```python
from build123d import *
from build123d.topology import SkipClean

# Parameters (mm, degrees)
SKETCH1_R           = 7.85
SKETCH1_R_2         = 3
BOSS_EXTRUDE1_DEPTH = 3
BOSS_EXTRUDE2_START = -6
BOSS_EXTRUDE2_DEPTH = 6
CUT_EXTRUDE1_DEPTH  = 1.5
CUT_EXTRUDE3_START  = -1.5
CUT_EXTRUDE3_DEPTH  = 1.5
SKETCH6_R           = 7.85
CUT_EXTRUDE4_DEPTH  = 1
SKETCH7_R           = 6.75
CUT_EXTRUDE5_DEPTH  = 4.2


with BuildPart() as part:
    # Sketch1 → Boss-Extrude1 (new, symmetric)
    # profile 1 of 7: a face of its own
    with BuildSketch(Plane(origin=(0, 0, 0), x_dir=(1, 0, 0), z_dir=(0, 1, 0))):
        with BuildLine():
            Line((10, 0), (7.85, 0))
            ThreePointArc((7.85, 0), (0, -7.85), (-7.85, 0))
            Line((-7.85, 0), (-101.897208147, 0))
            Line((-101.897208147, 0), (-112.298830122, -5.073262344))
            ThreePointArc((-112.298830122, -5.073262344), (-114.133881847, -5.566552555), (-116.020469414, -5.339534014))
            ThreePointArc((-116.020469414, -5.339534014), (-127.076790304, -20.864277212), (-109.083980094, -14.577890036))
            Line((-109.083980094, -14.577890036), (-90.484120267, -5.506038677))
            ThreePointArc((-90.484120267, -5.506038677), (-89.41701144, -5.128151962), (-88.292246268, -5))
            Line((-88.292246268, -5), (-11.180339887, -5))
            ThreePointArc((-11.180339887, -5), (-9.139098435, -5.435645354), (-7.453559925, -6.666666667))
            ThreePointArc((-7.453559925, -6.666666667), (3.568220898, -9.34172359), (10, 0))
        make_face()
        with Locations((-119.08, -14.86)):
            Circle(SKETCH1_R, mode=Mode.SUBTRACT)
    # profile 2 of 7: a face of its own
    with BuildSketch(Plane(origin=(0, 0, 0), x_dir=(1, 0, 0), z_dir=(0, 1, 0))):
        with Locations((-119.08, -14.86)):
            Circle(SKETCH1_R)
        with Locations(Location((-119.08, -14.86, 0), (0, 0, 270))):
            Circle(SKETCH1_R_2, mode=Mode.SUBTRACT)
    # profile 3 of 7: a face of its own
    with BuildSketch(Plane(origin=(0, 0, 0), x_dir=(1, 0, 0), z_dir=(0, 1, 0))):
        with BuildLine():
            ThreePointArc((-7.85, 0), (0, 7.85), (7.85, 0))
            Line((7.85, 0), (10, 0))
            ThreePointArc((10, 0), (3.568220898, 9.34172359), (-7.453559925, 6.666666667))
            ThreePointArc((-7.453559925, 6.666666667), (-9.139098435, 5.435645354), (-11.180339887, 5))
            Line((-11.180339887, 5), (-90.491443028, 5))
            ThreePointArc((-90.491443028, 5), (-91.616208201, 4.871848038), (-92.683317027, 4.493961323))
            Line((-92.683317027, 4.493961323), (-101.897208147, 0))
            Line((-101.897208147, 0), (-7.85, 0))
        make_face()
    # profile 4 of 7: a face of its own
    with BuildSketch(Plane(origin=(0, 0, 0), x_dir=(1, 0, 0), z_dir=(0, 1, 0))):
        with BuildLine():
            ThreePointArc((-3, 0), (0, 3), (3, 0))
            Line((3, 0), (7.85, 0))
            ThreePointArc((7.85, 0), (0, 7.85), (-7.85, 0))
            Line((-7.85, 0), (-3, 0))
        make_face()
    # profile 5 of 7: a face of its own
    with BuildSketch(Plane(origin=(0, 0, 0), x_dir=(1, 0, 0), z_dir=(0, 1, 0))):
        with BuildLine():
            Line((7.85, 0), (3, 0))
            ThreePointArc((3, 0), (0, -3), (-3, 0))
            Line((-3, 0), (-7.85, 0))
            ThreePointArc((-7.85, 0), (0, -7.85), (7.85, 0))
        make_face()
    # profile 6 of 7: a face of its own
    with BuildSketch(Plane(origin=(0, 0, 0), x_dir=(1, 0, 0), z_dir=(0, 1, 0))):
        with BuildLine():
            ThreePointArc((-3, 0), (0, 3), (3, 0))
            Line((3, 0), (7.85, 0))
            ThreePointArc((7.85, 0), (0, 7.85), (-7.85, 0))
            Line((-7.85, 0), (-3, 0))
        make_face()
    # profile 7 of 7: a face of its own
    with BuildSketch(Plane(origin=(0, 0, 0), x_dir=(1, 0, 0), z_dir=(0, 1, 0))):
        with BuildLine():
            Line((7.85, 0), (3, 0))
            ThreePointArc((3, 0), (0, -3), (-3, 0))
            Line((-3, 0), (-7.85, 0))
            ThreePointArc((-7.85, 0), (0, -7.85), (7.85, 0))
        make_face()
    extrude(amount=BOSS_EXTRUDE1_DEPTH, both=True)

    # Sketch3 → Boss-Extrude2 (add)
    with BuildSketch(Plane.XZ.offset(3).offset(BOSS_EXTRUDE2_START)):
        with BuildLine():
            Line((-109.083980094, 14.577890036), (-106.572243843, 13.352821776))
            ThreePointArc((-106.572243843, 13.352821776), (-108.334212899, 14.786207157), (-109.280246563, 16.851188733))
            ThreePointArc((-109.280246563, 16.851188733), (-109.117062064, 15.720155621), (-109.083980094, 14.577890036))
        make_face()
        with BuildLine():
            Line((-109.737977242, 15.328711334), (-109.083980094, 14.577890036))
            ThreePointArc((-109.083980094, 14.577890036), (-109.117062064, 15.720155621), (-109.280246563, 16.851188733))
            Line((-109.280246563, 16.851188733), (-109.737977242, 15.328711334))
        make_face()
    extrude(amount=BOSS_EXTRUDE2_DEPTH)

    # Sketch4 → Cut-Extrude1 (cut)
    with SkipClean():  # the faces are left unmerged after this step: merging them gives an invalid solid
        with BuildSketch(Plane(origin=(0, 3, 0), x_dir=(1, 0, 0), z_dir=(0, 1, 0))):
            with BuildLine():
                ThreePointArc((-7.453559925, 6.666666667), (-9.139098435, 5.435645354), (-11.180339887, 5))
                Line((-11.180339887, 5), (-90.491443028, 5))
                ThreePointArc((-90.491443028, 5), (-91.616208201, 4.871848038), (-92.683317027, 4.493961323))
                Line((-92.683317027, 4.493961323), (-112.298830122, -5.073262344))
                ThreePointArc((-112.298830122, -5.073262344), (-114.133881847, -5.566552555), (-116.020469414, -5.339534014))
                ThreePointArc((-116.020469414, -5.339534014), (-111.083209696, -8.855722788), (-109.083980094, -14.577890036))
                Line((-109.083980094, -14.577890036), (-106.572243843, -13.352821776))
                Line((-106.572243843, -13.352821776), (-90.484120267, -5.506038677))
                ThreePointArc((-90.484120267, -5.506038677), (-89.41701144, -5.128151962), (-88.292246268, -5))
                Line((-88.292246268, -5), (-11.180339887, -5))
                ThreePointArc((-11.180339887, -5), (-9.139098435, -5.435645354), (-7.453559925, -6.666666667))
                ThreePointArc((-7.453559925, -6.666666667), (-10, 0), (-7.453559925, 6.666666667))
            make_face()
            with BuildLine():
                Line((-106.572243843, -13.352821776), (-109.083980094, -14.577890036))
                ThreePointArc((-109.083980094, -14.577890036), (-109.080995073, -14.718930981), (-109.08, -14.86))
                ThreePointArc((-109.08, -14.86), (-109.13018758, -15.860616217), (-109.280246563, -16.851188733))
                ThreePointArc((-109.280246563, -16.851188733), (-108.334212899, -14.786207157), (-106.572243843, -13.352821776))
            make_face()
        extrude(amount=-CUT_EXTRUDE1_DEPTH, mode=Mode.SUBTRACT)

    # Sketch5 → Cut-Extrude3 (cut)
    with SkipClean():  # the faces are left unmerged after this step: merging them gives an invalid solid
        with BuildSketch(Plane.XZ.offset(3).offset(CUT_EXTRUDE3_START)):
            with BuildLine():
                ThreePointArc((-106.572243843, 13.352821776), (-108.334212899, 14.786207157), (-109.280246563, 16.851188733))
                ThreePointArc((-109.280246563, 16.851188733), (-109.13018758, 15.860616217), (-109.08, 14.86))
                ThreePointArc((-109.08, 14.86), (-109.080995073, 14.718930981), (-109.083980094, 14.577890036))
                Line((-109.083980094, 14.577890036), (-106.572243843, 13.352821776))
            make_face()
            with BuildLine():
                Line((-90.491443028, -5), (-11.180339887, -5))
                ThreePointArc((-11.180339887, -5), (-9.139098435, -5.435645354), (-7.453559925, -6.666666667))
                ThreePointArc((-7.453559925, -6.666666667), (-10, 0), (-7.453559925, 6.666666667))
                ThreePointArc((-7.453559925, 6.666666667), (-9.139098435, 5.435645354), (-11.180339887, 5))
                Line((-11.180339887, 5), (-88.292246268, 5))
                ThreePointArc((-88.292246268, 5), (-89.41701144, 5.128151962), (-90.484120267, 5.506038677))
                Line((-90.484120267, 5.506038677), (-106.572243843, 13.352821776))
                Line((-106.572243843, 13.352821776), (-109.083980094, 14.577890036))
                ThreePointArc((-109.083980094, 14.577890036), (-111.083209696, 8.855722788), (-116.020469414, 5.339534014))
                ThreePointArc((-116.020469414, 5.339534014), (-114.133881847, 5.566552555), (-112.298830122, 5.073262344))
                Line((-112.298830122, 5.073262344), (-92.683317027, -4.493961323))
                ThreePointArc((-92.683317027, -4.493961323), (-91.616208201, -4.871848038), (-90.491443028, -5))
            make_face()
        extrude(amount=CUT_EXTRUDE3_DEPTH, mode=Mode.SUBTRACT)

    # Sketch6 → Cut-Extrude4 (cut)
    with SkipClean():  # the faces are left unmerged after this step: merging them gives an invalid solid
        with BuildSketch(Plane(origin=(0, 3, 0), x_dir=(1, 0, 0), z_dir=(0, 1, 0))):
            with Locations(Location((-119.08, -14.86, 0), (0, 0, 270))):
                Circle(SKETCH6_R)
            with Locations(Location((0, 0, 0), (0, 0, 270))):
                Circle(SKETCH6_R)
        extrude(amount=-CUT_EXTRUDE4_DEPTH, mode=Mode.SUBTRACT)

    # Sketch7 → Cut-Extrude5 (cut)
    with SkipClean():  # the faces are left unmerged after this step: merging them gives an invalid solid
        with BuildSketch(Plane(origin=(0, 2, 0), x_dir=(1, 0, 0), z_dir=(0, 1, 0))):
            with Locations(Location((-119.08, -14.86, 0), (0, 0, 270))):
                Circle(SKETCH7_R)
            with Locations(Location((0, 0, 0), (0, 0, 270))):
                Circle(SKETCH7_R)
        extrude(amount=-CUT_EXTRUDE5_DEPTH, mode=Mode.SUBTRACT)


solid = part.part
```
Read the model definition and answer for the solid it produces. Units are mm, in the model's axes. A direction names the side the tool comes from. Round coordinates to 2 decimals unless told otherwise and drop trailing zeros. Write each loop counter-clockwise with the first axis right and the second up, starting at its lowest first coordinate (ties: lowest second). Pieces come first, ordered by that corner, then holes. Notation, with made-up numbers: (10.25, 19) -> (24.25, 19) arc R34 cw to (24.25, 51) -> close; hole circle Ø10 at (43.25, -3.5). An arc over 180 degrees is marked (long way). Answer in a Markdown table with one row per item. Add a question column.
1) Consider line 1 (Z direction, x = 0, y = -2.4); line 2 (X direction, y = -2.25, z = 15); line 3 (Z direction, x = -119.08, y = -2.75). Determine where each line is inside the solid, lowest interval first.
2) Find section C-C, the plane x = -34. Determine the outline of the cut face in (y, z), and give its area (3 significant figures).
3) Given P1, Ø3.5, axis at x = -52.5, y = -0.5, coming from the -Z side; P2, Ø1.5, axis at x = -42, y = 0, coming from the +Z side; P3, Ø3.5, axis at x = -119.08, z = 14.86, coming from the +Y side (3 decimals); P4, Ø7, axis at x = -1.5, z = 0, coming from the +Y side, each flat-ended and moving along its own axis, determine where each tip first touches the part or whether it passes through.
4) Find section B-B, the plane y = 0.25. Determine the outline of the cut face in (x, z).
5) Find section A-A, the plane x = 0. Determine the outline of the cut face in (y, z).
6) Which of the six approach directions +Z, -Z, +X, -X, +Y, -Y give full straight-line access (tool end or side, diameter ignored) to faces 5 (the face through (-4.777, 2.507, -6.229)), 6 (the face through (-50, 0, -5)), 7 (the face through (-89.43, -0.02, 5.13))?
7) Find section D-D, the plane z = 19.5. Determine the outline of the cut face in (x, y), and give its area (3 significant figures).
8) Determine the mould class of faces 1 (the face through (-113, 2, 11)), 2 (the face through (-91.601, -0.021, -4.875)), 3 (the face through (-1, -2.2, 3)), 4 (the face through (-62, 1.5, 2)) for opening direction Z: pulls with the +Z half, pulls with the -Z half, needs draft (parallel to the pull), parting line crosses it, or undercut.
Findings below:
| question | item | result |
|---|---|---|
| 1 | line 1 | -10 to -3, 3 to 10 |
| 1 | line 2 | -129.08 to -122.08, -116.08 to -109.08 |
| 1 | line 3 | 4.86 to 11.86, 17.86 to 24.86 |
| 2 | outline | (-1.5, -5) -> (1.5, -5) -> (1.5, 5) -> (-1.5, 5) -> close |
| 2 | area | 30.0 mm² |
| 3 | P1 | z = -5 |
| 3 | P2 | z = 5 |
| 3 | P3 | through |
| 3 | P4 | y = -2.2 |
| 4 | outline | (-116.02, 5.34) arc R5 cw to (-112.3, 5.07) -> (-92.68, -4.49) arc R5 ccw to (-90.49, -5) -> (-11.18, -5) arc R5 cw to (-7.45, -6.67) arc R10 ccw (long way) to (-7.45, 6.67) arc R5 cw to (-11.18, 5) -> (-88.29, 5) arc R5 cw to (-90.48, 5.51) -> (-106.57, 13.35) arc R5 cw to (-109.28, 16.85) arc R10 ccw (long way) to start; hole circle Ø13.5 at (-119.08, 14.86); hole circle Ø13.5 at (0, 0) |
| 5 | outline | (-3, -10) -> (3, -10) -> (3, -7.85) -> (2, -7.85) -> (2, -6.75) -> (-2.2, -6.75) -> (-2.2, -3) -> (-3, -3) -> close; (-3, 3) -> (-2.2, 3) -> (-2.2, 6.75) -> (2, 6.75) -> (2, 7.85) -> (3, 7.85) -> (3, 10) -> (-3, 10) -> close |
| 6 | face 5 | +Y |
| 6 | face 6 | -Z, -X, +Y, -Y |
| 6 | face 7 | +Z, +Y, -Y |
| 7 | outline | (-127.94, -3) -> (-110.22, -3) -> (-110.22, 3) -> (-112.75, 3) -> (-112.75, 2) -> (-114.18, 2) -> (-114.18, -2.2) -> (-123.98, -2.2) -> (-123.98, 2) -> (-125.41, 2) -> (-125.41, 3) -> (-127.94, 3) -> close |
| 7 | area | 52.5 mm² |
| 8 | face 1 | undercut |
| 8 | face 2 | pulls with the -Z half |
| 8 | face 3 | undercut |
| 8 | face 4 | needs draft |
